Read the model definition and answer for the solid it produces. Units are mm, in the model's axes. A direction names the side the tool comes from. Give positions to 0.01 mm unless a question says otherwise; leave off trailing zeros. Order: outer loops, then holes, each group sorted by start corner. A loop starts at its lowest first (then second) coordinate and runs counter-clockwise, first axis right, second up.
Item 1: A cutting plane is placed at C-C (x = -34.5). Write down the section's boundary in (y, z), plus the area to 3 significant figures.
Item 2: The mould has two halves that part along X. Classify faces 3 (the face through (-49.45, 49.33, 3.22)), 4 (the face through (16, 52, 0)): +X half, -X half, draft (parallel to the pull), parting line (faces both ways), or undercut.
Item 3: A cutting plane is placed at A-A (x = 0). Write down the section's boundary in (y, z).
Item 4: Which of the six approach directions +Z, -Z, +X, -X, +Y, -Y give full straight-line access (tool end or side, diameter ignored) to faces 1 (the face through (16, 52, 6.35)), 2 (the face through (-51.67, -42.69, 3.22))?
Item 5: Given pin 1 Ø1 at (y, z) = (-21.5, 5) entering from -X; pin 2 Ø1 at (x, z) = (-36, 4) entering from +Y; pin 3 Ø1.9 at (x, z) = (-57.5, 4) entering from +Y, each flat-ended and moving along its own axis, determine where each tip first touches the part or whether it passes through.
Item 6: A cutting plane is placed at D-D (y = -60). Write down the section's boundary in (x, z), plus the area to 3 significant figures.
Item 7: Find the intervals of material crossed by line 1 along Y through (x, z) = (0, 4.5); line 2 along Y through (x, z) = (41, 1); line 3 along Y through (x, z) = (-23.5, 2.5), in increasing order.
from build123d import *

# Parameters (mm, degrees)
SKETCH1_R           = 76.2
SKETCH1_R_2         = 53.086
BOSS_EXTRUDE2_DEPTH = 6.35
CUT_EXTRUDE1_REACH  = 109.95
SKETCH2_W           = 12.7
SKETCH2_H           = 6.35
CIRPATTERN1_COUNT   = 4
SPACER_HOLES_REACH  = 109.95
CIRPATTERN2_COUNT   = 4


with BuildPart() as part:
    # Sketch1 → Boss-Extrude2 (new body)
    with BuildSketch(Plane.XY):
        Circle(SKETCH1_R)
        Circle(SKETCH1_R_2, mode=Mode.SUBTRACT)
    extrude(amount=BOSS_EXTRUDE2_DEPTH)

    # Sketch2 → Cut-Extrude1 (cut, up to next)
    with BuildSketch(Plane.XY.offset(6.35), mode=Mode.PRIVATE) as cut_extrude1_sk1:
        with Locations((0, 70.4215)):
            Rectangle(SKETCH2_W, SKETCH2_H)
    cut_extrude1_tool1 = extrude(cut_extrude1_sk1.sketch, amount=-CUT_EXTRUDE1_REACH, mode=Mode.PRIVATE) & part.part
    # Sketch2 → Cut-Extrude1 (cut, up to next)
    with BuildSketch(Plane.XY.offset(6.35), mode=Mode.PRIVATE) as cut_extrude1_sk2:
        with Locations((0, 58.8645)):
            Rectangle(SKETCH2_W, SKETCH2_H)
    cut_extrude1_tool2 = extrude(cut_extrude1_sk2.sketch, amount=-CUT_EXTRUDE1_REACH, mode=Mode.PRIVATE) & part.part
    cut_extrude1_1 = cut_extrude1_tool1.solids().sort_by_distance((0, 70.4215, 6.35))[0]
    add(cut_extrude1_1, mode=Mode.SUBTRACT)
    cut_extrude1_2 = cut_extrude1_tool2.solids().sort_by_distance((0, 58.8645, 6.35))[0]
    add(cut_extrude1_2, mode=Mode.SUBTRACT)
    cut_extrude1 = cut_extrude1_1 + cut_extrude1_2  # Cut-Extrude1 as one shape, for the pattern or mirror that repeats it

    # CirPattern1: Cut-Extrude1 ×4 about axis
    cirpattern1_axis = Axis((0, 0, 0), (0, 0, 1))
    for i in range(1, CIRPATTERN1_COUNT):
        add(cut_extrude1.rotate(cirpattern1_axis, i * 360 / CIRPATTERN1_COUNT), mode=Mode.SUBTRACT)

    # Sketch3 → Spacer Holes (cut, up to next)
    with BuildSketch(Plane.XY.offset(6.35), mode=Mode.PRIVATE) as spacer_holes_sk1:
        Polygon((40.411152545, 49.391408666), (44.901280605, 53.881536726), (53.881536726, 44.901280605), (49.391408666, 40.411152545), align=None)
    spacer_holes_tool1 = extrude(spacer_holes_sk1.sketch, amount=-SPACER_HOLES_REACH, mode=Mode.PRIVATE) & part.part
    spacer_holes = spacer_holes_tool1.solids().sort_by_distance((47.146345, 47.146345, 6.35))[0]
    add(spacer_holes, mode=Mode.SUBTRACT)

    # CirPattern2: Spacer Holes ×4 about axis
    cirpattern2_axis = Axis((0, 0, 0), (0, 0, 1))
    for i in range(1, CIRPATTERN2_COUNT):
        add(spacer_holes.rotate(cirpattern2_axis, i * 360 / CIRPATTERN2_COUNT), mode=Mode.SUBTRACT)


solid = part.part
Response values:
1. outline: (-67.94, 0) - (-40.35, 0) - (-40.35, 6.35) - (-67.94, 6.35) - close; (40.35, 0) - (67.94, 0) - (67.94, 6.35) - (40.35, 6.35) - close
1. area: 350 mm2
2. face 3: undercut
2. face 4: draft
3. outline: (-76.2, 0) - (-73.6, 0) - (-73.6, 6.35) - (-76.2, 6.35) - close; (-67.25, 0) - (-62.04, 0) - (-62.04, 6.35) - (-67.25, 6.35) - close; (-55.69, 0) - (-53.09, 0) - (-53.09, 6.35) - (-55.69, 6.35) - close; (53.09, 0) - (55.69, 0) - (55.69, 6.35) - (53.09, 6.35) - close; (62.04, 0) - (67.25, 0) - (67.25, 6.35) - (62.04, 6.35) - close; (73.6, 0) - (76.2, 0) - (76.2, 6.35) - (73.6, 6.35) - close
4. face 1: +Z, +X, -X, +Y, -Y
4. face 2: +Z, -Z
5. pin 1: stops at x = -73.25
5. pin 2: stops at y = 67.43
5. pin 3: stops at y = 51.07
6. outline: (-46.97, 0) - (-6.35, 0) - (-6.35, 6.35) - (-46.97, 6.35) - close; (6.35, 0) - (46.97, 0) - (46.97, 6.35) - (6.35, 6.35) - close
6. area: 516 mm2
7. line 1: y = -76.2 to -73.6, -67.25 to -62.04, -55.69 to -53.09, 53.09 to 55.69, 62.04 to 67.25, 73.6 to 76.2
7. line 2: y = -64.23 to -49.98, -48.8 to -33.72, 33.72 to 48.8, 49.98 to 64.23
7. line 3: y = -72.49 to -47.6, 47.6 to 72.49
